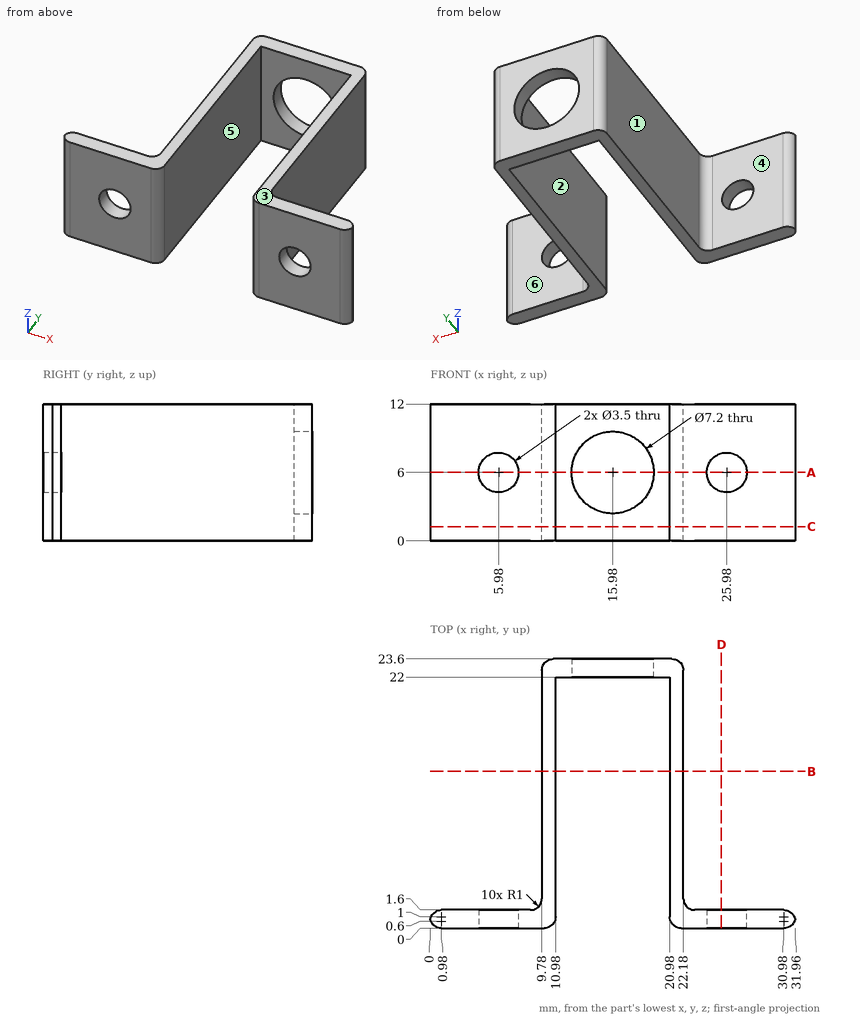
Input: dimensioned drawing with shaded views. Units: mm. Origin: part minimum x, y, z. A direction names the side the tool comes from. Coordinates: 2 decimals unless noted, no trailing zeros. Loops run counter-clockwise (first coordinate to the right, second up) from the corner with the lowest first, then second, coordinate; pieces in that order, holes last. Notation, with made-up numbers: M 17,70.5 L 49,70.5 A15 ccw 49,95.5 Z; hole C 13,-6 d3. An arc over 180 degrees is marked long. Use a Markdown table: item, result. Add a question column.
1) Set-up query: the marked faces 4, 5 and 6. Return all of +Z, -Z, +X, -X, +Y, -Y with unobstructed straight access to the full face (end or side cutting, diameter ignored); none if empty.
2) Draft query along X for the marked faces 1, 2 and 3. Return one class per face: +X half, -X half, draft (parallel to the pull), parting line (faces both ways), or undercut.
3) Section A-A, the plane z = 6. Give the number of separate pieces and of enclosed holes in the cut face.
4) Section D-D, the plane x = 25.5. Return the cut outline in (y, z).
5) Section C-C, the plane z = 1.25. Return the cut outline in (x, y).
6) Pin query (flat end, axial travel): P1, Ø3.5, axis at y = 15.5, z = 7, coming from the +X side; P2, Ø1, axis at x = 28.5, z = 5, coming from the +Y side; P3, Ø2, axis at y = 8, z = 8.5, coming from the -X side. Return the tip coordinate at first contact, or that it passes through.
7) Line query: L1, parallel to X at y = 7.25, z = 4.5; L2, parallel to Y at x = 24.5, z = 4.5; L3, parallel to Y at x = 11.5, z = 6.5. Output: solid intervals per line, ascending. Write a range as from..to.
8) Section B-B, the plane y = 13.75. Return the cut outline in (x, z).
Answer below:
| question | item | result |
|---|---|---|
| 1 | face 4 | +Z, -Z, -X, +Y |
| 1 | face 5 | +Z, -Z, -Y |
| 1 | face 6 | +Z, -Z, +X, +Y |
| 2 | face 1 | -X half |
| 2 | face 2 | undercut |
| 2 | face 3 | draft |
| 3 | separate pieces | 4 |
| 3 | enclosed holes | 0 |
| 4 | outline | M 0,0 L 1.6,0 L 1.6,4.32 L 0,4.32 Z; M 0,7.68 L 1.6,7.68 L 1.6,12 L 0,12 Z |
| 5 | outline | M 0,0.8 A1 ccw 0.98,0 L 9.98,0 A1 ccw 10.98,1 L 10.98,22 L 20.98,22 L 20.98,1 A1 ccw 21.98,0 L 30.98,0 A1 ccw 31.96,0.8 A1 ccw 30.98,1.6 L 23.18,1.6 A1 cw 22.18,2.6 L 22.18,22.6 A1 ccw 21.18,23.6 L 10.78,23.6 A1 ccw 9.78,22.6 L 9.78,2.6 A1 cw 8.78,1.6 L 0.98,1.6 A1 ccw Z |
| 6 | P1 | x = 22.18 |
| 6 | P2 | y = 1.6 |
| 6 | P3 | x = 9.78 |
| 7 | L1 | 9.78..10.98, 20.98..22.18 |
| 7 | L2 | 0..1.6 |
| 7 | L3 | 22..23.6 |
| 8 | outline | M 9.78,0 L 10.98,0 L 10.98,12 L 9.78,12 Z; M 20.98,0 L 22.18,0 L 22.18,12 L 20.98,12 Z |
